```python
from build123d import *

# Parameters (mm, degrees)
SKETCH_1_W          = 20
SKETCH_1_H          = 40
EXTRUDE_1_DEPTH     = 27
SKETCH_2_W          = 20
SKETCH_2_H          = 54
EXTRUDE_2_DEPTH     = 2.5
SKETCH_3_W          = 20
SKETCH_3_H          = 40
EXTRUDE_3_DEPTH     = 8
SKETCH_4_R          = 2
CUT_EXTRUDE_1_DEPTH = 42.221960167
SKETCH_5_R          = 10
EXTRUDE_4_DEPTH     = 4
SKETCH_6_R          = 2.9
EXTRUDE_5_DEPTH     = 3.6


with BuildPart() as part:
    # 草图1 → 凸台-拉伸1 (new body)
    with BuildSketch(Plane(origin=(0, 0, 0), x_dir=(1, 0, 0), z_dir=(0, 1, 0))):
        Rectangle(SKETCH_1_W, SKETCH_1_H)
    extrude(amount=EXTRUDE_1_DEPTH)

    # 草图2 → 凸台-拉伸2 (add)
    with BuildSketch(Plane(origin=(0, 27, 0), x_dir=(1, 0, 0), z_dir=(0, 1, 0))):
        Rectangle(SKETCH_2_W, SKETCH_2_H)
    extrude(amount=EXTRUDE_2_DEPTH)

    # 草图3 → 凸台-拉伸3 (add)
    with BuildSketch(Plane(origin=(0, 29.5, 0), x_dir=(1, 0, 0), z_dir=(0, 1, 0))):
        Rectangle(SKETCH_3_W, SKETCH_3_H)
    extrude(amount=EXTRUDE_3_DEPTH)

    # 草图4 → 切除-拉伸1 (cut, through all)
    with BuildSketch(Plane(origin=(0, 29.5, 0), x_dir=(1, 0, 0), z_dir=(0, 1, 0))):
        with Locations(Location((-5, -24.3, 0), (0, 0, 270))):
            Circle(SKETCH_4_R)
        with Locations(Location((5, -24.3, 0), (0, 0, 270))):
            Circle(SKETCH_4_R)
        with Locations(Location((-5, 24.3, 0), (0, 0, 270))):
            Circle(SKETCH_4_R)
        with Locations(Location((5, 24.3, 0), (0, 0, 270))):
            Circle(SKETCH_4_R)
    extrude(amount=-CUT_EXTRUDE_1_DEPTH, mode=Mode.SUBTRACT)

    # 草图5 → 凸台-拉伸4 (add)
    with BuildSketch(Plane(origin=(0, 37.5, 0), x_dir=(1, 0, 0), z_dir=(0, 1, 0))):
        with Locations(Location((0, 10, 0), (0, 0, 90))):
            Circle(SKETCH_5_R)
    extrude(amount=EXTRUDE_4_DEPTH)

    # 草图6 → 凸台-拉伸5 (add)
    with BuildSketch(Plane(origin=(0, 41.5, 0), x_dir=(1, 0, 0), z_dir=(0, 1, 0))):
        with Locations(Location((0, 10, 0), (0, 0, 270))):
            Circle(SKETCH_6_R)
    extrude(amount=EXTRUDE_5_DEPTH)


solid = part.part
```
Geometry check sheet. Reference: the model listing, model coordinates, mm. A direction names the side the tool comes from. Round coordinates to 2 decimals unless told otherwise and drop trailing zeros. Order: outer loops, then holes, each group sorted by start corner. A loop starts at its lowest first (then second) coordinate and runs counter-clockwise, first axis right, second up. Notation, with made-up numbers: (-9, -12.5) -> (-1, -12.5) arc R22 ccw to (-1, -0.5) -> close; hole circle Ø7 at (87, 36). An arc over 180 degrees is marked (long way). Return JSON: item names as keys, results as strings. Group by question number.
Q1. Section check C-C, the plane y = 28.5. Record the boundary of the cut face in (x, z).
Q2. Release check for a two-part mould opening along Z. For faces 4 (the flat face through (8, 37.5, -18)), 5 (the cylindrical face through (-4.912, 28.268, 22.302)), 6 (the flat face through (0, 13, -20)) record: released by +Z, released by -Z, zero draft, split by the parting line, or undercut.
Q3. Tool access check on faces 1 (the flat face through (0, 29.5, -24)), 2 (the flat face through (0, 27, 23)), 3 (the cylindrical face through (0, 39, 0)). Record the directions out of +Z, -Z, +X, -X, +Y, -Y that give a thin tool (end or side, any length) a straight path to the whole face; none if there is none.
Q4. Section check B-B, the plane x = 5. Record the boundary of the cut face in (y, z), plus the area to 3 significant figures.
Q5. Section check A-A, the plane z = 24.3. Record the boundary of the cut face in (x, y).
Q6. Material ranges on probe 1 along X at (y, z) = (28.5, 24.3); probe 2 along Y at (x, z) = (1.25, 15); probe 3 along Z at (x, y) = (0.25, 21.5), recorded low to high. Write a range as from..to.
Q7. Gauge pin test, flat ends, axial feed: pin 1 (2 mm diameter, centred on x = -3, z = 23.5, fed in from -Y); pin 2 (5 mm diameter, centred on x = -5, z = 24.3, fed in from +Y); pin 3 (3 mm diameter, centred on x = -2, y = 22.5, fed in from -Z); pin 4 (3 mm diameter, centred on x = -5, z = -24.3, fed in from +Y). Record the tip position at first contact, or that the pin passes through.
Q8. Section check D-D, the plane z = -16. Record the boundary of the cut face in (x, y).
Numbers:
{
 "1": {"outline": "(-10, -27) -> (10, -27) -> (10, 27) -> (-10, 27) -> close; hole circle Ø4 at (-5, -24.3); hole circle Ø4 at (-5, 24.3); hole circle Ø4 at (5, -24.3); hole circle Ø4 at (5, 24.3)"},
 "2": {"face 4": "zero draft", "face 5": "undercut", "face 6": "released by -Z"},
 "3": {"face 1": "-Z, +X, -X, +Y", "face 2": "+Z, +X, -X, -Y", "face 3": "+Y"},
 "4": {"outline": "(0, -20) -> (27, -20) -> (27, -22.3) -> (29.5, -22.3) -> (29.5, -20) -> (37.5, -20) -> (37.5, -18.66) -> (41.5, -18.66) -> (41.5, -1.34) -> (37.5, -1.34) -> (37.5, 20) -> (29.5, 20) -> (29.5, 22.3) -> (27, 22.3) -> (27, 20) -> (0, 20) -> close; (27, -27) -> (29.5, -27) -> (29.5, -26.3) -> (27, -26.3) -> close; (27, 26.3) -> (29.5, 26.3) -> (29.5, 27) -> (27, 27) -> close", "area": "1,580 mm^2"},
 "5": {"outline": "(-10, 27) -> (-7, 27) -> (-7, 29.5) -> (-10, 29.5) -> close; (-3, 27) -> (3, 27) -> (3, 29.5) -> (-3, 29.5) -> close; (7, 27) -> (10, 27) -> (10, 29.5) -> (7, 29.5) -> close"},
 "6": {"probe 1": "-10..-7, -3..3, 7..10", "probe 2": "0..37.5", "probe 3": "-20..20"},
 "7": {"pin 1": "y = 27", "pin 2": "y = 29.5", "pin 3": "z = -20", "pin 4": "through"},
 "8": {"outline": "(-10, 0) -> (10, 0) -> (10, 37.5) -> (8, 37.5) -> (8, 41.5) -> (-8, 41.5) -> (-8, 37.5) -> (-10, 37.5) -> close"}
}
